```python
from build123d import *

# Parameters (mm, degrees)
F0_W     = 12.6746
F0_H     = 9.525
F0_W_2   = 0.0508
F1_DEPTH = 3.175
F2_DEPTH = 6.35


with BuildPart() as f1:
    # F0 (on Top) → F1 (new body)
    with BuildSketch(Plane.XY):
        with Locations((-6.3627, 4.7625)):
            Rectangle(F0_W, F0_H)
        with Locations((6.3627, 4.7625)):
            Rectangle(F0_W, F0_H)
        with Locations((6.3627, -4.7625)):
            Rectangle(F0_W, F0_H)
        with Locations((-6.3627, -4.7625)):
            Rectangle(F0_W, F0_H)
        with Locations((0, 4.7625)):
            Rectangle(F0_W_2, F0_H)
        with Locations((0, -4.7625)):
            Rectangle(F0_W_2, F0_H)
    extrude(amount=F1_DEPTH)

    # F0 (on Top) → F2 (join)
    with BuildSketch(Plane.XY):
        with Locations((6.3627, -4.7625)):
            Rectangle(F0_W, F0_H)
        with Locations((-6.3627, 4.7625)):
            Rectangle(F0_W, F0_H)
    extrude(amount=F2_DEPTH)


solid = f1.part
```
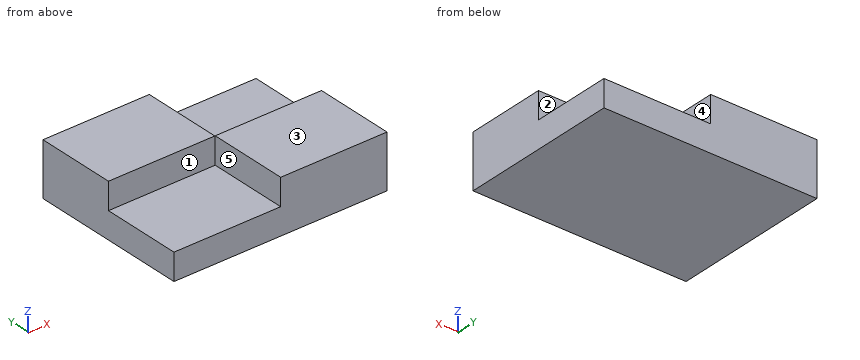
For this review, take the finished solid that the model builds, in its own axes (mm). Face numbers are marked on the shaded views. A direction names the side the tool comes from. Coordinates: 2 decimals unless noted, no trailing zeros. Loops run counter-clockwise (first coordinate to the right, second up) from the corner with the lowest first, then second, coordinate; pieces in that order, holes last.
1. For line 1 (Y direction, x = -2.5, z = 4) (3 decimals); line 2 (Y direction, x = 1.5, z = 5.5) (3 decimals); line 3 (X direction, y = 2.25, z = 4), list the stretches that pass through material, from the lowest coordinate up.
2. For the marked faces 1, 2, 3, 4 and 5, list the 3-axis set-ups (+Z, -Z, +X, -X, +Y, -Y) from which the entire face can be reached by the end or side of a thin tool; tool diameter is ignored.
3. Insertion check: P1, Ø3, axis at x = -5.5, y = -1.5, coming from the -Z side; P2, Ø2.5, axis at x = -4.5, z = 5, coming from the -Y side; P3, Ø1.6, axis at x = 9, z = 5, coming from the +Y side; P4, Ø3.5, axis at y = -2.5, z = 5, coming from the -X side. Each pin has a flat end and moves straight along its axis. Give the tip position at first contact, or say it passes through.
4. Add section A-A, the plane z = 3.5. Give the boundary of the cut face in (x, y) (3 decimals).
5. Add section C-C, the plane x = 4. Give the boundary of the cut face in (y, z) (3 decimals).
6. Add section B-B, the plane y = -4.75. Give the boundary of the cut face in (x, z) (3 decimals).
Result:
1. line 1: y = 0 to 9.525
1. line 2: y = -9.525 to 0
1. line 3: x = -12.7 to -0.03
2. face 1: +Z, -X, -Y
2. face 2: +Z, +X, +Y
2. face 3: +Z, +X, -X, +Y, -Y
2. face 4: +Z, +X, +Y, -Y
2. face 5: +Z, -X, +Y, -Y
3. P1: stops at z = 0
3. P2: stops at y = 0
3. P3: stops at y = 0
3. P4: stops at x = 0.03
4. outline: (-12.7, 0) - (-0.025, 0) - (-0.025, 9.525) - (-12.7, 9.525) - close; (0.025, -9.525) - (12.7, -9.525) - (12.7, 0) - (0.025, 0) - close
5. outline: (-9.525, 0) - (9.525, 0) - (9.525, 3.175) - (0, 3.175) - (0, 6.35) - (-9.525, 6.35) - close
6. outline: (-12.7, 0) - (12.7, 0) - (12.7, 6.35) - (0.025, 6.35) - (0.025, 3.175) - (-12.7, 3.175) - close
